Model file for the job. Use its own axes, mm. Face numbers are marked on the shaded views. A direction names the side the tool comes from. Coordinates: 2 decimals unless noted, no trailing zeros. Order: outer loops, then holes, each group sorted by start corner. A loop starts at its lowest first (then second) coordinate and runs counter-clockwise, first axis right, second up. Notation, with made-up numbers: M 27,-4.5 L 56,-4.5 A19 ccw 56,17.5 Z; hole C -10,-17.5 d10. An arc over 180 degrees is marked long. Return JSON: item names as keys, results as strings.
```python
from build123d import *

# Parameters (mm, degrees)
EXTRUDE_THIN1_DEPTH     = 50
SKETCH2_R               = 7.5
CUT_EXTRUDE1_DEPTH      = 33.5
CUT_EXTRUDE1_DEPTH_BACK = 33.5
FILLET1_R               = 5


with BuildPart() as part:
    # Sketch1 → Extrude-Thin1 (new body, symmetric)
    with BuildSketch(Plane(origin=(0, 0, 0), x_dir=(0, 0, -1), z_dir=(1, 0, 0))):
        Polygon((-27.5, -50), (-27.5, 0), (27.5, 0), (27.5, -50), (32.5, -50), (32.5, 5), (-32.5, 5), (-32.5, -50), align=None)
    extrude(amount=EXTRUDE_THIN1_DEPTH, both=True)

    # Sketch2 → Cut-Extrude1 (cut, two sides)
    with BuildSketch(Plane.XY) as cut_extrude1_sk:
        with Locations((-25, -25)):
            Circle(SKETCH2_R)
        with Locations((25, -25)):
            Circle(SKETCH2_R)
    extrude(amount=CUT_EXTRUDE1_DEPTH, mode=Mode.SUBTRACT)
    extrude(cut_extrude1_sk.sketch, amount=-CUT_EXTRUDE1_DEPTH_BACK, mode=Mode.SUBTRACT)

    # Fillet1
    fillet1_edges = [part.edges().sort_by_distance(p)[0] for p in [
        (50, -50, 30),
        (50, -50, -30),
        (-50, -50, 30),
        (-50, -50, -30),
    ]]
    fillet(fillet1_edges, radius=FILLET1_R)


solid = part.part
```
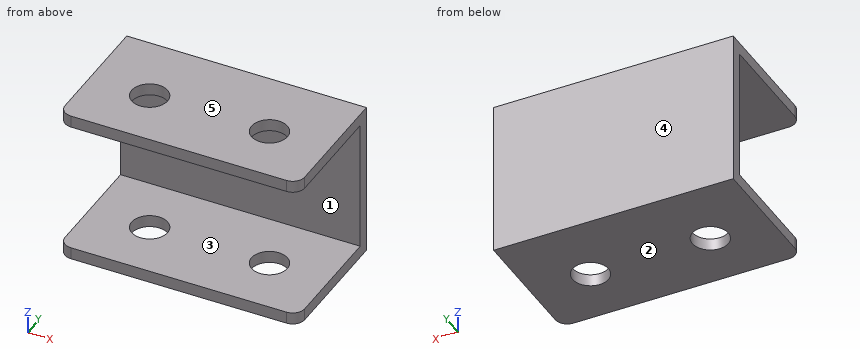
Item 1: Pull direction Z, two halves, no side cores. Call the marked faces 3, 4 and 5: +Z half, -Z half, draft (parallel to the pull), parting line (faces both ways), or undercut.
Check result:
{"face 3": "undercut", "face 4": "draft", "face 5": "+Z half"}
Item 2: Saw through at C-C (y = -5). Write the cut outline in (x, z).
Check result:
{"outline": "M -50,-32.5 L 50,-32.5 L 50,-27.5 L -50,-27.5 Z; M -50,27.5 L 50,27.5 L 50,32.5 L -50,32.5 Z"}
Item 3: Saw through at B-B (y = -25). Write the cut outline in (x, z).
Check result:
{"outline": "M -50,-32.5 L -32.5,-32.5 L -32.5,-27.5 L -50,-27.5 Z; M -50,27.5 L -32.5,27.5 L -32.5,32.5 L -50,32.5 Z; M -17.5,-32.5 L 17.5,-32.5 L 17.5,-27.5 L -17.5,-27.5 Z; M -17.5,27.5 L 17.5,27.5 L 17.5,32.5 L -17.5,32.5 Z; M 32.5,-32.5 L 50,-32.5 L 50,-27.5 L 32.5,-27.5 Z; M 32.5,27.5 L 50,27.5 L 50,32.5 L 32.5,32.5 Z"}
Item 4: Saw through at D-D (x = -25). Write the cut outline in (y, z), and give its area (3 significant figures).
Check result:
{"outline": "M -50,-32.5 L -32.5,-32.5 L -32.5,-27.5 L -50,-27.5 Z; M -50,27.5 L -32.5,27.5 L -32.5,32.5 L -50,32.5 Z; M -17.5,-32.5 L 5,-32.5 L 5,32.5 L -17.5,32.5 L -17.5,27.5 L 0,27.5 L 0,-27.5 L -17.5,-27.5 Z", "area": "675 mm2"}
Item 5: Drop flat-ended pins along their axis: pin 1 Ø5 at (x, z) = (-30, 15) entering from -Y; pin 2 Ø13.5 at (x, y) = (25, -25) entering from -Z; pin 3 Ø24 at (x, y) = (-25, -25) entering from -Z. Give the stop position or say it passes through.
Check result:
{"pin 1": "stops at y = 0", "pin 2": "passes through", "pin 3": "stops at z = -32.5"}
Item 6: 3-axis set-ups, long thin cutter, end or side, ignore diameter. For the marked faces 1 and 2: which of +Z, -Z, +X, -X, +Y, -Y reach the whole face in a straight line?
Check result:
{"face 1": "+X, -X, -Y", "face 2": "-Z, +X, -X, +Y, -Y"}
Item 7: Saw through at A-A (x = 29.5). Write the cut outline in (y, z).
Check result:
{"outline": "M -50,-32.5 L -31,-32.5 L -31,-27.5 L -50,-27.5 Z; M -50,27.5 L -31,27.5 L -31,32.5 L -50,32.5 Z; M -19,-32.5 L 5,-32.5 L 5,32.5 L -19,32.5 L -19,27.5 L 0,27.5 L 0,-27.5 L -19,-27.5 Z"}
Item 8: Wall check: line 1 (X direction, y = -25, z = 30.5); line 2 (Z direction, x = 15, y = -4.5); line 3 (Y direction, x = -25, z = -30). Give the ranges that are in metal, low to high.
Check result:
{"line 1": "x = -50 to -32.5, -17.5 to 17.5, 32.5 to 50", "line 2": "z = -32.5 to -27.5, 27.5 to 32.5", "line 3": "y = -50 to -32.5, -17.5 to 5"}
